Check sheet for the modelled part. Datum: model origin and axes. Units: mm. Face numbers are marked on the shaded views. A direction names the side the tool comes from. Round coordinates to 2 decimals unless told otherwise and drop trailing zeros. Write each loop counter-clockwise with the first axis right and the second up, starting at its lowest first coordinate (ties: lowest second). Pieces come first, ordered by that corner, then holes. Notation, with made-up numbers: (86, 17.5) -> (131, 17.5) arc R20 ccw to (131, 43.5) -> close; hole circle Ø3 at (62.5, 26.25). An arc over 180 degrees is marked (long way). One line per item, written item: value.
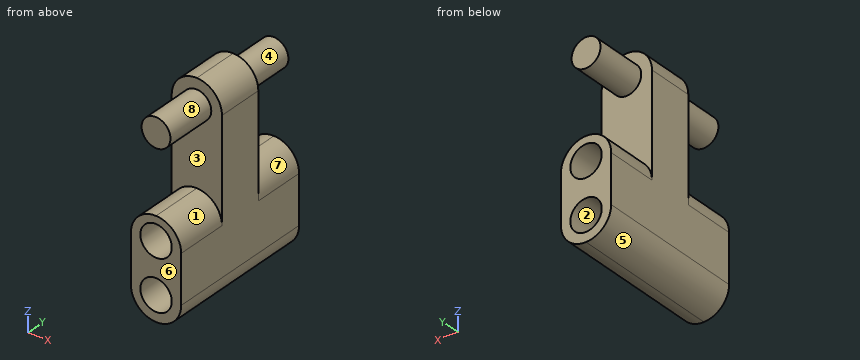
Autodesk Inventor part; units mm, degrees
ref_plane "YZ Plane" through (0, 0, 0) normal (1, 0, 0) x (0, 1, 0)
ref_plane "XZ Plane" through (0, 0, 0) normal (0, 1, 0) x (-1, 0, 0)
ref_plane "XY Plane" through (0, 0, 0) normal (0, 0, 1) x (1, 0, 0)
sketch "Sketch1" plane through (0, 0, 0) normal (0, 1, 0) x (-1, 0, 0)
  line L0 (0, 0) -> (-8, 0)
  line L1 (-8, 0) -> (-8, -15.7)
  line L2 (-8, -15.7) -> (0, -15.7)
  line L3 (0, -15.7) -> (0, 0)
  circle A0 centre (-4, -3.7) radius 2.5
  circle A1 centre (-4, -11.7) radius 2.5
  dimension "d0" = 8
  dimension "d1" = 15.7
  dimension "d4" = 5
  dimension "d5" = 5
  dimension "d8" = 8
  dimension "d15" = 4
extrude "Extrusion1" add sketch "Sketch1" along normal blind 24
fillet "Fillet1" radius 4 2 edges at (8, 12, 0) (0, 12, 0)
fillet "Fillet2" radius 4 2 edges at (8, 12, -15.7) (0, 12, -15.7)
sketch "Sketch2" plane through (0, 0, -4) normal (-1, 0, 0) x (0, 0, 1)
  line L0 (0, 8.3) -> (20.3, 8.3)
  line L1 (20.3, 8.3) -> (20.3, 15.7)
  line L2 (20.3, 15.7) -> (0, 15.7)
  line L3 (0, 15.7) -> (0, 8.3)
  line L4 (0, 24) -> (4, 24)
  line L5 (0, 24) -> (0, 0)
  point P0 (4, 0)
  dimension "d17" = 20.3
  dimension "d18" = 7.4
  dimension "d19" = 8.3
extrude "Extrusion2" add sketch "Sketch2" against normal blind 8
sketch "Sketch4" plane through (0, 15.7, 16.3) normal (0, 1, 0) x (1, 0, 0)
  circle A0 centre (4, 4) radius 2.3
  line L0 (8, 20.3) -> (8, 0)
  line L1 (0, 0) -> (8, 0)
  point P0 (0, 16.3)
  point P1 (8, 12)
  dimension "d24" = 4.6
  dimension "d25" = 4
  dimension "d26" = 4
extrude "Extrusion4" add sketch "Sketch4" along normal blind 8.3 and the other way blind 15.7
fillet "Fillet3" radius 4 2 edges at (0, 12, 16.3) (8, 12, 16.3)
sketch "Sketch5" plane through (4, 15.7, -3.7) normal (0, 1, 0) x (1, 0, 0)
  circle A0 centre (0, 0) radius 2.5
  point P0 (-4, -3.7)
extrude "Extrusion5" cut sketch "Sketch5" against normal through all
properties part number "Crank0"
Item 1: Sectioned sample at B-B (x = 5.5). Enter the section's corners in (y, z).
Result set:
outline: (0, -15.41) -> (24, -15.41) -> (24, -13.7) -> (0, -13.7) -> close; (0, -9.7) -> (24, -9.7) -> (24, -5.7) -> (0, -5.7) -> close; (0, -1.7) -> (24, -1.7) -> (24, -0.29) -> (15.7, -0.29) -> (15.7, 10.56) -> (24, 10.56) -> (24, 14.04) -> (15.7, 14.04) -> (15.7, 16.01) -> (8.3, 16.01) -> (8.3, 14.04) -> (0, 14.04) -> (0, 10.56) -> (8.3, 10.56) -> (8.3, -0.29) -> (0, -0.29) -> close
Item 2: Material ranges on line 1 along Z through (x, y) = (4, 3.25); line 2 along Z through (x, y) = (4, 15.5); line 3 along Z through (x, y) = (4.5, 18) (3 decimals), recorded low to high.
Result set:
line 1: -15.7 to -14.2, -9.2 to -6.2, -1.2 to 0, 10 to 14.6
line 2: -15.7 to -14.2, -9.2 to -6.2, -1.2 to 16.3
line 3: -15.669 to -14.149, -9.251 to -6.149, -1.251 to -0.031, 10.055 to 14.545
Item 3: Sectioned sample at C-C (z = 11). Enter the section's corners in (x, y), then the cut area to 3 significant figures.
Result set:
outline: (0, 8.3) -> (2.1, 8.3) -> (2.1, 0) -> (5.9, 0) -> (5.9, 8.3) -> (8, 8.3) -> (8, 15.7) -> (5.9, 15.7) -> (5.9, 24) -> (2.1, 24) -> (2.1, 15.7) -> (0, 15.7) -> close
area: 122 mm^2
Item 4: Depth check by flat-ended pin: pin 1 (2.5 mm diameter, centred on x = 4, z = 1.5, fed in from +Y); pin 2 (3 mm diameter, centred on x = 6, z = -10.5, fed in from +Y); pin 3 (4 mm diameter, centred on x = 5, z = 7, fed in from -Y); pin 4 (1.5 mm diameter, centred on x = 2.5, y = 17.5, fed in from +Z). Enter the tip coordinate at first touch or a pass-through.
Result set:
pin 1: y = 15.7
pin 2: y = 24
pin 3: y = 8.3
pin 4: z = 14.47
Item 5: Sectioned sample at A-A (z = -5.5). Enter the section's corners in (x, y).
Result set:
outline: (0, 0) -> (2.27, 0) -> (2.27, 24) -> (0, 24) -> close; (5.73, 0) -> (8, 0) -> (8, 24) -> (5.73, 24) -> close
Item 6: Release check for a two-part mould opening along X. For the marked faces 1, 2 and 3 record: pulls with the +X half, pulls with the -X half, needs draft (parallel to the pull), parting line crosses it, or undercut.
Result set:
face 1: pulls with the +X half
face 2: undercut
face 3: needs draft
Item 7: Sectioned sample at D-D (x = 3). Enter the section's corners in (y, z).
Result set:
outline: (0, -15.57) -> (24, -15.57) -> (24, -13.99) -> (0, -13.99) -> close; (0, -9.41) -> (24, -9.41) -> (24, -5.99) -> (0, -5.99) -> close; (0, -1.41) -> (24, -1.41) -> (24, -0.13) -> (15.7, -0.13) -> (15.7, 10.23) -> (24, 10.23) -> (24, 14.37) -> (15.7, 14.37) -> (15.7, 16.17) -> (8.3, 16.17) -> (8.3, 14.37) -> (0, 14.37) -> (0, 10.23) -> (8.3, 10.23) -> (8.3, -0.13) -> (0, -0.13) -> close
Item 8: Tool access check on the marked faces 4, 5, 6, 7 and 8. Record the directions out of +Z, -Z, +X, -X, +Y, -Y that give a thin tool (end or side, any length) a straight path to the whole face; none if there is none.
Result set:
face 4: +Y
face 5: -Z, -X, +Y, -Y
face 6: +Z, -Z, +X, -X, -Y
face 7: +X, +Y
face 8: -Y
